from build123d import *

# Parameters (mm, degrees)
PAD_DEPTH       = 50
POCKET_DEPTH    = 18.001
SKETCH003_R     = 10.6
POCKET001_DEPTH = 30.3
SKETCH004_R     = 10.6
POCKET002_DEPTH = 30.3
SKETCH005_R     = 1.65
SKETCH005_R_2   = 2.65
POCKET007_DEPTH = 18.001
POCKET008_DEPTH = 5
SKETCH006_R     = 1.25
POCKET009_DEPTH = 10
CHAMFER_SIZE    = 2


with BuildPart() as part:
    # Sketch001 → Pad (new body, symmetric)
    with BuildSketch(Plane.XZ):
        with BuildLine():
            Line((-20.5, 0), (-6.5, 0))
            ThreePointArc((-6.5, 0), (0, -6.5), (6.5, 0))
            Line((6.5, 0), (20.5, 0))
            Line((20.5, 0), (20.5, -18))
            Line((20.5, -18), (-120.5, -18))
            Line((-120.5, -18), (-120.5, -13))
            Line((-20.5, -13), (-120.5, -13))
            Line((-20.5, 0), (-20.5, -13))
        make_face()
    extrude(amount=PAD_DEPTH, both=True)

    # Sketch002 → Pocket (cut, through all)
    with BuildSketch(Plane.XY):
        Polygon((-20.5, 50), (-120.5, 50), (-120.5, -30), align=None)
    extrude(amount=-POCKET_DEPTH, mode=Mode.SUBTRACT)

    # Sketch003 (on DatumPlane) → Pocket001 (cut)
    with BuildSketch(Plane.XZ.offset(45)):
        Circle(SKETCH003_R)
    extrude(amount=-POCKET001_DEPTH, mode=Mode.SUBTRACT)

    # Sketch004 (on DatumPlane) → Pocket002 (cut)
    with BuildSketch(Plane.XZ.offset(-45)):
        Circle(SKETCH004_R)
    extrude(amount=POCKET002_DEPTH, mode=Mode.SUBTRACT)

    # Sketch005 → Pocket007 (cut, through all)
    with BuildSketch(Plane.XY):
        with Locations((-15.5, -40)):
            Circle(SKETCH005_R)
        with Locations((15.5, -40)):
            Circle(SKETCH005_R)
        with Locations((15.5, 0)):
            Circle(SKETCH005_R)
        with Locations((15.5, 40)):
            Circle(SKETCH005_R)
        with Locations((-15.5, 40)):
            Circle(SKETCH005_R)
        with Locations((-15.5, 0)):
            Circle(SKETCH005_R)
        with Locations((-110.5, -40)):
            Circle(SKETCH005_R_2)
        with Locations((-70.5, -40)):
            Circle(SKETCH005_R_2)
        with Locations((-30.5, -40)):
            Circle(SKETCH005_R_2)
    extrude(amount=-POCKET007_DEPTH, mode=Mode.SUBTRACT)

    # Sketch (on DatumPlane) → Pocket008 (cut)
    with BuildSketch(Plane.XY.offset(-18)):
        Polygon((-12.75, 38.412287), (-12.75, 41.587713), (-15.5, 43.175426), (-18.25, 41.587713), (-18.25, 38.412287), (-15.5, 36.824574), align=None)
        Polygon((18.25, 38.412287), (18.25, 41.587713), (15.5, 43.175426), (12.75, 41.587713), (12.75, 38.412287), (15.5, 36.824574), align=None)
        Polygon((-12.75, -1.587713), (-12.75, 1.587713), (-15.5, 3.175426), (-18.25, 1.587713), (-18.25, -1.587713), (-15.5, -3.175426), align=None)
        Polygon((18.25, -1.587713), (18.25, 1.587713), (15.5, 3.175426), (12.75, 1.587713), (12.75, -1.587713), (15.5, -3.175426), align=None)
        Polygon((-12.75, -41.587713), (-12.75, -38.412287), (-15.5, -36.824574), (-18.25, -38.412287), (-18.25, -41.587713), (-15.5, -43.175426), align=None)
        Polygon((18.25, -41.587713), (18.25, -38.412287), (15.5, -36.824574), (12.75, -38.412287), (12.75, -41.587713), (15.5, -43.175426), align=None)
    extrude(amount=POCKET008_DEPTH, mode=Mode.SUBTRACT)

    # Sketch006 (on DatumPlane) → Pocket009 (cut)
    with BuildSketch(Plane.YZ.offset(20.5)):
        with Locations((-45, -8)):
            Circle(SKETCH006_R)
        with Locations((-10, -8)):
            Circle(SKETCH006_R)
        with Locations((10, -8)):
            Circle(SKETCH006_R)
        with Locations((45, -8)):
            Circle(SKETCH006_R)
    extrude(amount=-POCKET009_DEPTH, mode=Mode.SUBTRACT)

    # Chamfer
    chamfer_edges = [part.edges().sort_by_distance(p)[0] for p in [
        (-20.5, 0, -13),
    ]]
    chamfer(chamfer_edges, length=CHAMFER_SIZE)


solid = part.part
Geometry: final body of the model. Coordinates: model frame, mm. A direction names the side the tool comes from. Give positions to 0.01 mm unless a question says otherwise; leave off trailing zeros. Loops run counter-clockwise (first coordinate to the right, second up) from the corner with the lowest first, then second, coordinate; pieces in that order, holes last. Notation, with made-up numbers: (26, 3) - (80, 3) arc R30 ccw to (80, 37) - close; hole circle Ø2 at (-20.75, 10.5). An arc over 180 degrees is marked (long way). Answer as CSV lines item,"result". Start each with the question number.
1. Section A-A, the plane y = 0. Return loops of the section in (x, z), plus the area to 3 significant figures.
2. Reachability of faces 1 (the face through (-60, -12, -13)), 2 (the face through (-13.976, -0.632, -6.409)), 3 (the face through (16.86, 37.61, -15.54)) from +Z, -Z, +X, -X, +Y, -Y: full face, straight path, thin tool, end or side. Return the list, or none.
3. Ray query, L1, parallel to Y at x = 10.5, z = -0.75; L2, parallel to Y at x = 15.5, z = -4; L3, parallel to X at y = 4, z = -7.25. Return the intervals inside material, ascending.
4. Section D-D, the plane x = -30.5. Return loops of the section in (y, z).
5. Draft query along X for faces 4 (the face through (18.25, -40, -16)), 5 (the face through (0, 14.7, -8)), 6 (the face through (-120.5, -40, -16)), 7 (the face through (0, 50, -9)). Return one class per face: released by +X, released by -X, zero draft, split by the parting line, or undercut.
6. Pin query (flat end, axial travel): P1, Ø3, axis at y = -10, z = -8, coming from the -X side; P2, Ø1.2, axis at y = -9.5, z = -8, coming from the +X side; P3, Ø3, axis at x = 14.5, y = 40, coming from the -Z side; P4, Ø4, axis at x = -30.5, y = -40, coming from the +Z side. Return the tip coordinate at first contact, or that it passes through.
7. Section C-C, the plane z = -3. Give the number of separate pieces and of enclosed holes in the cut face, plus the area to 3 significant figures.
8. Section B-B, the plane x = -70.5. Return loops of the section in (y, z).
Answers:
1,outline,"(-83, -18) - (-18.25, -18) - (-18.25, -13) - (-17.15, -13) - (-17.15, 0) - (-20.5, 0) - (-20.5, -11) - (-22.5, -13) - (-83, -13) - close; (-13.85, -13) - (-12.75, -13) - (-12.75, -18) - (12.75, -18) - (12.75, -13) - (13.85, -13) - (13.85, 0) - (6.5, 0) arc R6.5 cw to (-6.5, 0) - (-13.85, 0) - close; (17.15, -13) - (18.25, -13) - (18.25, -18) - (20.5, -18) - (20.5, 0) - (17.15, 0) - close"
1,area,"845 mm2"
2,face 1,"+Z, -X, +Y, -Y"
2,face 2,"+Z, -Z"
2,face 3,"-Z"
3,L1,"y = -50 to -45, -14.7 to 14.7, 45 to 50"
3,L2,"y = -50 to -41.65, -38.35 to -1.65, 1.65 to 38.35, 41.65 to 50"
3,L3,"x = -20.5 to 20.5"
4,outline,"(-50, -18) - (-42.65, -18) - (-42.65, -13) - (-50, -13) - close; (-37.35, -18) - (42, -18) - (42, -13) - (-37.35, -13) - close"
5,face 4,"undercut"
5,face 5,"undercut"
5,face 6,"released by -X"
5,face 7,"zero draft"
6,P1,"stops at x = -20.5"
6,P2,"stops at x = 10.5"
6,P3,"stops at z = -13"
6,P4,"passes through"
7,separate pieces,"2"
7,enclosed holes,"6"
7,area,"2,360 mm2"
8,outline,"(-50, -18) - (-42.65, -18) - (-42.65, -13) - (-50, -13) - close; (-37.35, -18) - (10, -18) - (10, -13) - (-37.35, -13) - close"
